The listing builds one solid part. Answer for the finished solid, in the listing's coordinates (mm). Face numbers are marked on the shaded views. A direction names the side the tool comes from. Coordinates: 2 decimals unless noted, no trailing zeros. Write each loop counter-clockwise with the first axis right and the second up, starting at its lowest first coordinate (ties: lowest second). Pieces come first, ordered by that corner, then holes.
from build123d import *

# Parameters (mm, degrees)
F0_W     = 5.5
F0_H     = 2
F1_DEPTH = 15
F2_W     = 2
F2_H     = 11
F3_DEPTH = 13.501
F4_W     = 2
F4_H     = 2
F5_DEPTH = 13.5
F6_R     = 2
F7_SIZE  = 0.5


with BuildPart() as f1:
    # F0 (on Top) → F1 (new body)
    with BuildSketch(Plane.XY):
        Polygon((29.5, -1), (27.5, -1), (22, -1), (6, -1), (0, -1), (0, -3), (29.5, -3), align=None)
        with Locations((24.75, 0)):
            Rectangle(F0_W, F0_H)
        Polygon((27.5, 1), (27.5, -1), (29.5, -1), (29.5, 10.5), (27.5, 10.5), align=None)
        Polygon((29.5, 10.5), (29.5, -1), (33.5, -1), (33.5, 12.5), (29.5, 12.5), align=None)
        Polygon((0, -1), (6, -1), (6, 1), (-6, 1), (-6, -1), align=None)
        Polygon((25.5, 10.5), (27.5, 10.5), (29.5, 10.5), (29.5, 12.5), (27.5, 12.5), (25.5, 11.5), align=None)
        Polygon((0, -3), (0, -1), (-6, -1), (-22, -1), (-27.5, -1), (-29.5, -1), (-29.5, -3), align=None)
        with Locations((-24.75, 0)):
            Rectangle(F0_W, F0_H)
        Polygon((-29.5, 10.5), (-29.5, -1), (-27.5, -1), (-27.5, 1), (-27.5, 10.5), align=None)
        Polygon((-33.5, -1), (-29.5, -1), (-29.5, 10.5), (-29.5, 12.5), (-33.5, 12.5), align=None)
        Polygon((-29.5, 12.5), (-29.5, 10.5), (-27.5, 10.5), (-25.5, 10.5), (-25.5, 11.5), (-27.5, 12.5), align=None)
    extrude(amount=F1_DEPTH)

    # F2 (on face) → F3 (cut, through all)
    with BuildSketch(Plane.XZ.offset(1)):
        with Locations((-30.5, 7.5)):
            Rectangle(F2_W, F2_H)
        with Locations((30.5, 7.5)):
            Rectangle(F2_W, F2_H)
    extrude(amount=-F3_DEPTH, mode=Mode.SUBTRACT)

    # F4 (on face) → F5 (join)
    with BuildSketch(Plane.XY.offset(15)):
        with Locations((-6.5, -4)):
            Rectangle(F4_W, F4_H)
        Polygon((7.5, -7), (7.5, -3), (5.5, -3), (5.5, -5), (-5.5, -5), (-7.5, -5), (-7.5, -7), align=None)
    extrude(amount=-F5_DEPTH)

    # F6
    f6_edges = [f1.edges().sort_by_distance(p)[0] for p in [
        (33.5, 5.75, 15),
        (-33.5, 5.75, 15),
        (33.5, 5.75, 0),
        (-33.5, 5.75, 0),
        (-27.5, 12.5, 7.5),
        (27.5, 12.5, 7.5),
        (-7.5, -7, 8.25),
        (7.5, -7, 8.25),
    ]]
    fillet(f6_edges, radius=F6_R)

    # F7
    f7_edges = [f1.edges().sort_by_distance(p)[0] for p in [
        (-31.5, -1, 7.5),
        (-30.5, -1, 13),
        (-30.5, -1, 2),
        (31.5, -1, 7.5),
        (30.5, -1, 13),
        (30.5, -1, 2),
        (31.5, 12.5, 7.5),
        (30.5, 12.5, 2),
        (29.5, 12.5, 7.5),
        (30.5, 12.5, 13),
        (-30.5, 12.5, 2),
        (-29.5, 12.5, 7.5),
        (-31.5, 12.5, 7.5),
        (-30.5, 12.5, 13),
        (0, -3, 15),
        (-5.5, -4, 15),
        (0, -5, 15),
        (5.5, -4, 15),
    ]]
    chamfer(f7_edges, length=F7_SIZE)


solid = f1.part
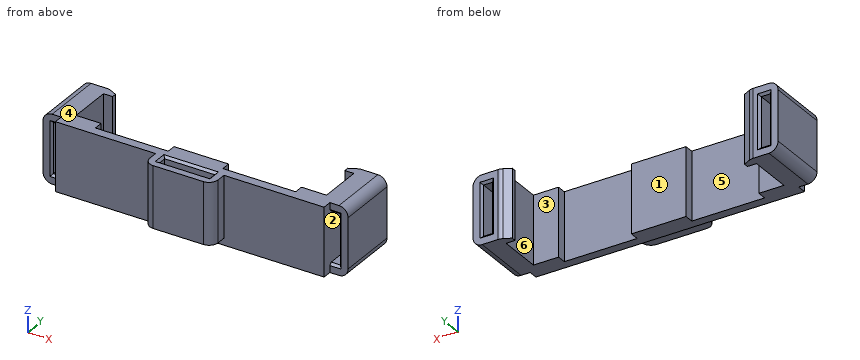
1. Flat-ended cylindrical pins translate along their axes: P1, Ø9, axis at x = -1.5, z = 6.5, coming from the +Y side; P2, Ø1, axis at y = -4, z = 11, coming from the +X side; P3, Ø4, axis at x = -25.5, z = 2, coming from the -Y side. Find the tip coordinate at first contact, or state that the pin passes through.
Results found:
P1: stops at y = 1
P2: stops at x = 7.5
P3: stops at y = -3
2. Section C-C on y = -3.75 is taken. Give the vertices of the cut face in (x, z), then the cut area to 4 significant figures.
Results found:
outline: (-7.5, 1.5) - (-5.5, 1.5) - (-5.5, 14.5) - (-6, 15) - (-7.5, 15) - close; (5.5, 1.5) - (7.5, 1.5) - (7.5, 15) - (6, 15) - (5.5, 14.5) - close
area: 53.75 mm2
3. Section A-A on y = 4.25 is taken. Give the vertices of the cut face in (x, z), then the cut area to 3 significant figures.
Results found:
outline: (-33.5, 2) arc R2 ccw to (-31.5, 0) - (-27.5, 0) - (-27.5, 15) - (-31.5, 15) arc R2 ccw to (-33.5, 13) - close; (27.5, 0) - (31.5, 0) arc R2 ccw to (33.5, 2) - (33.5, 13) arc R2 ccw to (31.5, 15) - (27.5, 15) - close; hole (-31.5, 2) - (-29.5, 2) - (-29.5, 13) - (-31.5, 13) - close; hole (29.5, 2) - (31.5, 2) - (31.5, 13) - (29.5, 13) - close
area: 133 mm2
4. For a pull along Y with two mould halves and no side action, classify the marked faces 1, 2 and 3 as pulls with the +Y half, pulls with the -Y half, needs draft (parallel to the pull), parting line crosses it, or undercut.
Results found:
face 1: pulls with the +Y half
face 2: needs draft
face 3: undercut
5. A tool of negligible diameter and unlimited length cuts with its end or side. For the marked faces 4, 5 and 6, from which of +Z, -Z, +X, -X, +Y, -Y can it reach the whole face along a straight path? Write none if from no direction.
Results found:
face 4: +Z, +X, -X, +Y, -Y
face 5: +Z, -Z, +Y
face 6: +Z, -Z
6. Section D-D on z = 10 is taken. State how many separate pieces and enclosed holes the cut face has, then the cut area to 4 significant figures.
Results found:
separate pieces: 3
enclosed holes: 1
area: 313.5 mm2
7. Section B-B on y = 0.25 is taken. Give the vertices of the cut face in (x, z).
Results found:
outline: (-33.5, 2) arc R2 ccw to (-31.5, 0) - (-22, 0) - (-22, 15) - (-31.5, 15) arc R2 ccw to (-33.5, 13) - close; (-6, 0) - (6, 0) - (6, 15) - (-6, 15) - close; (22, 0) - (31.5, 0) arc R2 ccw to (33.5, 2) - (33.5, 13) arc R2 ccw to (31.5, 15) - (22, 15) - close; hole (-31.5, 2) - (-29.5, 2) - (-29.5, 13) - (-31.5, 13) - close; hole (29.5, 2) - (31.5, 2) - (31.5, 13) - (29.5, 13) - close
8. Find the intervals of material crossed by L1, parallel to X at y = 0.25, z = 6; L2, parallel to X at y = 8, z = 2.25; L3, parallel to Z at x = -30.5, y = 10.75, in increasing order.
Results found:
L1: x = -33.5 to -31.5, -29.5 to -22, -6 to 6, 22 to 29.5, 31.5 to 33.5
L2: x = -33.5 to -31.5, -29.5 to -27.5, 27.5 to 29.5, 31.5 to 33.5
L3: z = 0 to 2, 13 to 15
